Check sheet for the modelled part. Datum: model origin and axes. Units: mm. Face numbers are marked on the shaded views. A direction names the side the tool comes from. Round coordinates to 2 decimals unless told otherwise and drop trailing zeros. Order: outer loops, then holes, each group sorted by start corner. A loop starts at its lowest first (then second) coordinate and runs counter-clockwise, first axis right, second up.
```python
from build123d import *

# Parameters (mm, degrees)
SKETCH_3_R          = 14
EXTRUDE_2_DEPTH     = 7
CUT_EXTRUDE_1_DEPTH = 8
SKETCH_10_W         = 12
SKETCH_10_H         = 18
CUT_EXTRUDE_2_DEPTH = 2
SKETCH_12_R         = 0.8
CUT_EXTRUDE_3_DEPTH = 11.5


with BuildPart() as part:
    # Эскиз3 → Бобышка-Вытянуть2 (new body)
    with BuildSketch(Plane(origin=(0, 0, 0), x_dir=(1, 0, 0), z_dir=(0, 1, 0))):
        Circle(SKETCH_3_R)
    extrude(amount=EXTRUDE_2_DEPTH)

    # Эскиз8 → Вырез-Вытянуть1 (cut, through all)
    with BuildSketch(Plane(origin=(0, 7, 0), x_dir=(1, 0, 0), z_dir=(0, 1, 0))):
        Polygon((-2.5, 10.977260976), (-2.5, 10), (2.5, 10), (2.5, -10), (-1.5, -10), (-1.5, -11), (-5.5, -11), (-5.5, -6), (-10.5, -6), (-10.5, 6), (-5.5, 6), (-5.5, 10.977260976), align=None)
    extrude(amount=-CUT_EXTRUDE_1_DEPTH, mode=Mode.SUBTRACT)

    # Эскиз10 → Вырез-Вытянуть2 (cut)
    with BuildSketch(Plane(origin=(0, 7, 0), x_dir=(1, 0, 0), z_dir=(0, 1, 0))):
        with Locations((4.25, 0)):
            Rectangle(SKETCH_10_W, SKETCH_10_H)
    extrude(amount=-CUT_EXTRUDE_2_DEPTH, mode=Mode.SUBTRACT)

    # Эскиз12 → Вырез-Вытянуть3 (cut)
    with BuildSketch(Plane(origin=(14, 0, 0), x_dir=(0, 0, -1), z_dir=(1, 0, 0))):
        with Locations((0, 2.5)):
            Circle(SKETCH_12_R)
    extrude(amount=-CUT_EXTRUDE_3_DEPTH, mode=Mode.SUBTRACT)


solid = part.part
```
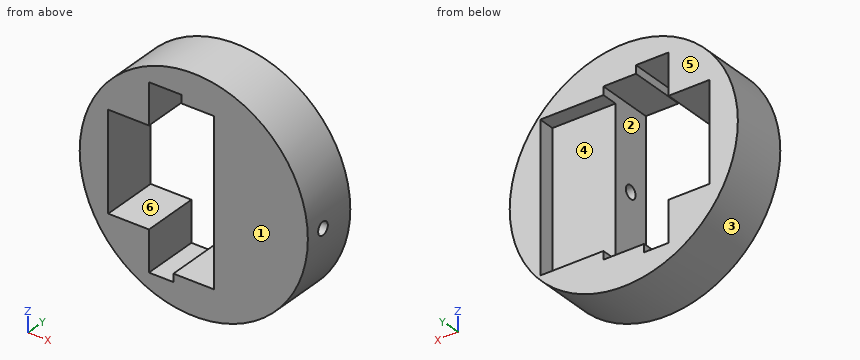
Item 1: Sectioned sample at A-A (z = 0). Record the cut outline in (x, y), and give its area (3 significant figures).
Answer:
outline: (-14, 0) - (-10.5, 0) - (-10.5, 7) - (-14, 7) - close; (2.5, 0) - (14, 0) - (14, 1.7) - (2.5, 1.7) - close; (2.5, 3.3) - (14, 3.3) - (14, 7) - (10.25, 7) - (10.25, 5) - (2.5, 5) - close
area: 71.1 mm2
Item 2: Sectioned sample at D-D (z = 4.5). Record the cut outline in (x, y).
Answer:
outline: (-13.26, 0) - (-10.5, 0) - (-10.5, 7) - (-13.26, 7) - close; (2.5, 0) - (13.26, 0) - (13.26, 7) - (10.25, 7) - (10.25, 5) - (2.5, 5) - close
Item 3: Access from +Z, -Z, +X, -X, +Y, -Y to the whole of each face (thin tool, end or side, straight path). Record for the marked faces 4, 5 and 6.
Answer:
face 4: +Y
face 5: +Z, -Z, +X, -X, +Y
face 6: +Y, -Y
Item 4: Sectioned sample at B-B (x = 0). Record the cut outline in (y, z), and give its area (3 significant figures).
Answer:
outline: (0, -14) - (7, -14) - (7, -10) - (0, -10) - close; (0, 10) - (7, 10) - (7, 14) - (0, 14) - close
area: 56.0 mm2
Item 5: Scan lines: line 1 along Y through (x, z) = (11, 0); line 2 along X through (y, z) = (5.75, 0); line 3 along Y through (x, z) = (7.5, 0). Record each from-to range of solid material in increasing order.
Answer:
line 1: y = 0 to 1.7, 3.3 to 7
line 2: x = -14 to -10.5, 10.25 to 14
line 3: y = 0 to 1.7, 3.3 to 5
Item 6: Sectioned sample at C-C (y = 6). Record the cut outline in (x, z).
Answer:
outline: circle Ø28 at (0, 0); hole (-10.5, -6) - (-5.5, -6) - (-5.5, -10.98) - (-2.5, -10.98) - (-2.5, -10) - (2.5, -10) - (2.5, -9) - (10.25, -9) - (10.25, 9) - (2.5, 9) - (2.5, 10) - (-1.5, 10) - (-1.5, 11) - (-5.5, 11) - (-5.5, 6) - (-10.5, 6) - close
Item 7: Go/stop test with flat-tipped pins: P1, Ø2, axis at x = -7, y = 1.5, coming from the +Z side; P2, Ø1.5, axis at x = 2.5, y = 2.5, coming from the +Z side; P3, Ø2.5, axis at x = 7.5, z = -2.5, coming from the +Y side. Record where each tip stops, or that it passes through.
Answer:
P1: stops at z = 12.65
P2: stops at z = 13.89
P3: stops at y = 5
Item 8: Release check for a two-part mould opening along X. For the marked faces 1, 2 and 3 record: released by +X, released by -X, zero draft, split by the parting line, or undercut.
Answer:
face 1: zero draft
face 2: undercut
face 3: split by the parting line
